Here's the drawing with two shaded views (mm, measured from the low corner). I have some questions. Round coordinates to 2 decimals unless told otherwise and drop trailing zeros. Order: outer loops, then holes, each group sorted by start corner. A loop starts at its lowest first (then second) coordinate and runs counter-clockwise, first axis right, second up. Notation, with made-up numbers: M 22,-25.75 L 38,-25.75 A30 cw 38,13.25 Z; hole C 63.25,-6.75 d4. An arc over 180 degrees is marked long. One line per question, with ' | ' between items.
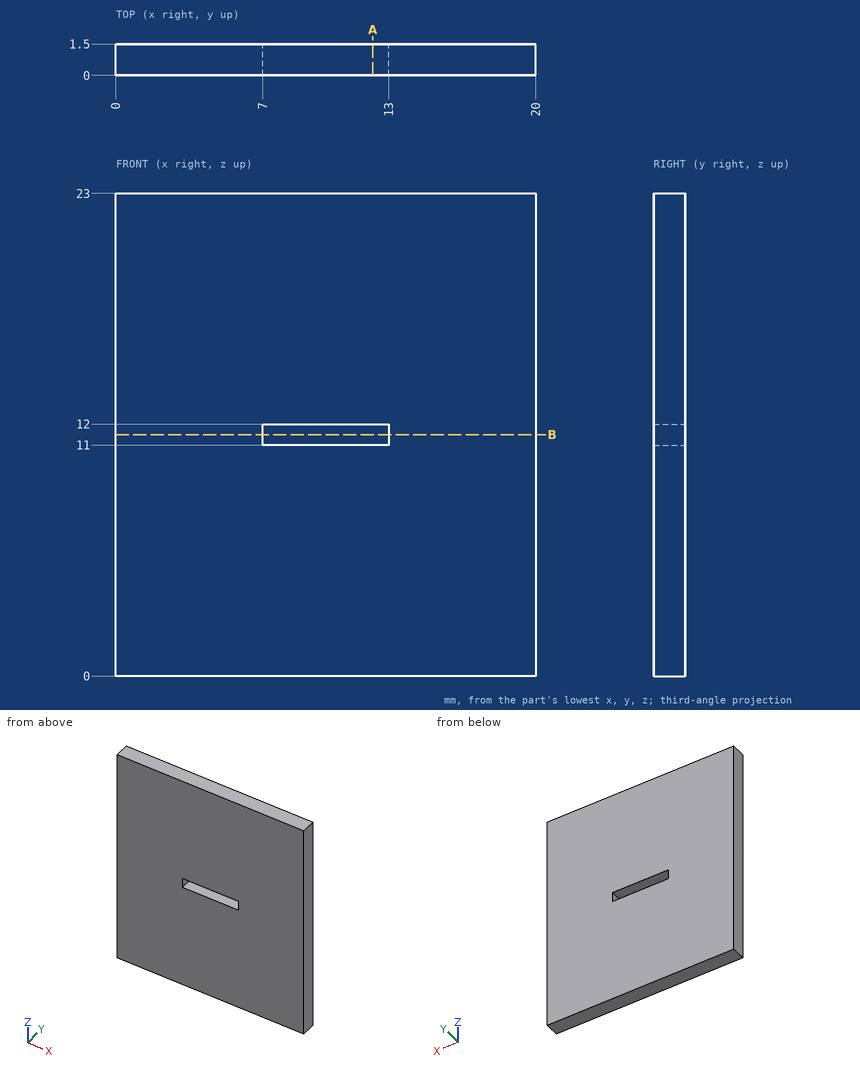
(1) Please list where these lines run through material, in increasing order: probe 1 along Z at (x, y) = (12.25, 0.7); probe 2 along X at (y, z) = (0.95, 11.75). Write a range as [from, to].
Final values:
probe 1: [0, 11], [12, 23] | probe 2: [0, 7], [13, 20]
(2) If we section it at A-A on x = 12.25: Please give me the cut outline in (y, z), plus the area to 3 significant figures.
Final values:
outline: M 0,0 L 1.5,0 L 1.5,11 L 0,11 Z; M 0,12 L 1.5,12 L 1.5,23 L 0,23 Z | area: 33.0 mm^2
(3) If we section it at B-B on z = 11.5: Please give me the cut outline in (x, y).
Final values:
outline: M 0,0 L 7,0 L 7,1.5 L 0,1.5 Z; M 13,0 L 20,0 L 20,1.5 L 13,1.5 Z
